from build123d import *

# Parameters (mm, degrees)
F4_DEPTH    = 11
F5_T1_DEPTH = 41
F5_T3_DEPTH = 40.0473750966
F6_R        = 6
F7_T        = -2.5
F8_W        = 56.25
F8_H        = 2.5
F9_DEPTH    = 8.5
F11_DEPTH   = 8.5
F12_R       = 5
F13_DEPTH   = 56.25


# Not quite as in the source:
# - a fillet or chamfer that OpenCascade refuses, or shapes differently, is made with other operations: its cross-section is extruded or revolved along the edge and cut away or added


with BuildPart() as f4:
    # F3 (on Top) → F4 (new body)
    with BuildSketch(Plane.XY):
        Polygon((-35.5, 33.75), (-35.5, -48.75), (35.5, -48.75), (35.5, 33.75), (40, 33.75), (40, 48.75), (-40, 48.75), (-40, 33.75), align=None)
    extrude(amount=F4_DEPTH)

    # F5: fillet of radius 6 on 6 edges, made by hand

    # F5_s2 → F5_t1 (cut)
    with BuildSketch(Plane.XY.offset(-15)):
        with BuildLine():
            ThreePointArc((-35.5, -42.75), (-33.7426406871, -46.9926406871), (-29.5, -48.75))
            Line((-29.5, -48.75), (-35.5, -48.75))
            Line((-35.5, -48.75), (-35.5, -42.75))
        make_face()
        with BuildLine():
            ThreePointArc((29.5, -48.75), (33.7426406871, -46.9926406871), (35.5, -42.75))
            Line((35.5, -42.75), (35.5, -48.75))
            Line((35.5, -48.75), (29.5, -48.75))
        make_face()
        with BuildLine():
            ThreePointArc((40, 42.75), (38.2426406871, 46.9926406871), (34, 48.75))
            Line((34, 48.75), (40, 48.75))
            Line((40, 48.75), (40, 42.75))
        make_face()
        with BuildLine():
            ThreePointArc((-34, 48.75), (-38.2426406871, 46.9926406871), (-40, 42.75))
            Line((-40, 42.75), (-40, 48.75))
            Line((-40, 48.75), (-34, 48.75))
        make_face()
    extrude(amount=F5_T1_DEPTH, mode=Mode.SUBTRACT)

    # F5_s4 → F5_t3 (cut)
    with BuildSketch(Plane.XY.offset(-14.5236875483)):
        with BuildLine():
            ThreePointArc((-40, 39.5594750193), (-38.7434164903, 35.8852404051), (-35.5, 33.75))
            Line((-35.5, 33.75), (-40, 33.75))
            Line((-40, 33.75), (-40, 39.5594750193))
        make_face()
        with BuildLine():
            ThreePointArc((35.5, 33.75), (38.7434164903, 35.8852404051), (40, 39.5594750193))
            Line((40, 39.5594750193), (40, 33.75))
            Line((40, 33.75), (35.5, 33.75))
        make_face()
    extrude(amount=F5_T3_DEPTH, mode=Mode.SUBTRACT)

    # F6
    f6_edges = [f4.edges().sort_by_distance(p)[0] for p in [
        (35.5, 33.75, 5.5),
        (-35.5, 33.75, 5.5),
    ]]
    fillet(f6_edges, radius=F6_R)

    # F7
    f7_openings = [f4.faces().sort_by_distance(p)[0] for p in [
        (0, 0.742075, 11),
    ]]
    offset(amount=F7_T, openings=f7_openings)

    # F8 (on face) → F9 (cut)
    with BuildSketch(Plane.XY.offset(11)):
        with Locations((0, 47.5)):
            Rectangle(F8_W, F8_H)
    extrude(amount=-F9_DEPTH, mode=Mode.SUBTRACT)

    # F10 (on face) → F11 (join)
    with BuildSketch(Plane.XY.offset(2.5)):
        Polygon((-28.125, 48.75), (-28.125, 46.25), (-28.125, 35), (28.125, 35), (28.125, 48.75), (26.875, 48.75), (26.875, 36.25), (-26.875, 36.25), (-26.875, 48.75), align=None)
    extrude(amount=F11_DEPTH)

    # F12 (on face) → F13 (cut)
    with BuildSketch(Plane(origin=(-28.125, 0, 0), x_dir=(0, -1, 0), z_dir=(-1, 0, 0))):
        with Locations((-41.25, 11)):
            Circle(F12_R)
    extrude(amount=-F13_DEPTH, mode=Mode.SUBTRACT)


solid = f4.part
For this review, take the finished solid that the model builds, in its own axes (mm). A direction names the side the tool comes from. Give positions to 0.01 mm unless a question says otherwise; leave off trailing zeros. Order: outer loops, then holes, each group sorted by start corner. A loop starts at its lowest first (then second) coordinate and runs counter-clockwise, first axis right, second up. Notation, with made-up numbers: M 88,-19 L 136,-19 A21 cw 136,5 Z; hole C 60.5,-17.5 d10. An arc over 180 degrees is marked long. Answer in a Markdown table with one row per item. Add a question column.
(1) Consider section B-B on y = -15.5. State the section outline as (x, z) points.
(2) Mouldability with a two-part tool opening along Y and no side actions: class faces 4 (the face through (33.696, -47.039, 5.423)), 5 (the face through (-40, 41, 5)), 6 (the face through (-37.164, 38.064, 6.69)) as +Y half, -Y half, draft (parallel to the pull), parting line (faces both ways), or undercut.
(3) Wall thickness on probe 1 along X at (y, z) = (-8.5, 7.25); probe 2 along Y at (x, z) = (-21.5, 3.25); probe 3 along Z at (x, y) = (-14.5, -23): over which ranges is each line inside the solid? List them lowest first. Write a range as [from, to].
(4) Consider section A-A on x = -9.5. State the section outline as (y, z) points.
(5) For faces 1 (the face through (0, -48.75, 5)), 2 (the face through (31.9, -45.3, 6.7)), 3 (the face through (0, 43, 2.5)), list the 3-axis set-ups (+Z, -Z, +X, -X, +Y, -Y) from which the entire face can be reached by the end or side of a thin tool; tool diameter is ignored.
(6) Consider section C-C on y = 41.25. State the section outline as (x, z) points (3 decimals), and give its area (3 significant figures).
(7) For pin 1 (6.5 mm diameter, centred on x = 30, z = 6.5, fed in from -Y); pin 2 (1.5 mm diameter, centred on x = 8.5, y = -7.5, fed in from +Z); pin 3 (3 mm diameter, centred on x = -32.5, z = 6.5, fed in from -Y); pin 4 (2 mm diameter, centred on y = 27, z = 4, fed in from +X), all flat-tipped, find the tip position at first contact; note any pin that passes through.
Evaluation:
| question | item | result |
|---|---|---|
| 1 | outline | M -35.5,0 L 35.5,0 L 35.5,11 L 33,11 L 33,2.5 L -33,2.5 L -33,11 L -35.5,11 Z |
| 2 | face 4 | -Y half |
| 2 | face 5 | draft |
| 2 | face 6 | undercut |
| 3 | probe 1 | x = [-35.5, -33], [33, 35.5] |
| 3 | probe 2 | y = [-48.75, -46.25], [35, 36.25] |
| 3 | probe 3 | z = [0, 2.5] |
| 4 | outline | M -48.75,0 L 48.75,0 L 48.75,2.5 L 36.25,2.5 L 36.25,11 L 35,11 L 35,2.5 L -46.25,2.5 L -46.25,11 L -48.75,11 Z |
| 5 | face 1 | +Z, -Z, +X, -X, -Y |
| 5 | face 2 | +Z |
| 5 | face 3 | +Z, +Y |
| 6 | outline | M -40,0 L 40,0 L 40,11 L 37.5,11 L 37.5,2.5 L 28.125,2.5 L 28.125,6 L 26.875,6 L 26.875,2.5 L -26.875,2.5 L -26.875,6 L -28.125,6 L -28.125,2.5 L -37.5,2.5 L -37.5,11 L -40,11 Z |
| 6 | area | 251 mm^2 |
| 7 | pin 1 | stops at y = -48.75 |
| 7 | pin 2 | stops at z = 2.5 |
| 7 | pin 3 | stops at y = -48.56 |
| 7 | pin 4 | stops at x = 35.5 |
